The listing builds one solid part. Answer for the finished solid, in the listing's coordinates (mm). Round coordinates to 2 decimals unless told otherwise and drop trailing zeros. Write each loop counter-clockwise with the first axis right and the second up, starting at its lowest first coordinate (ties: lowest second). Pieces come first, ordered by that corner, then holes.
(1) A cutting plane is placed at D-D, the plane y = 1.75. Give the number of separate pieces and of enclosed holes in the cut face, and give its area (3 significant figures).
(2) A cutting plane is placed at B-B, the plane z = 0. Give the vertices of the cut face in (x, y).
(3) Find the intervals of material crossed by probe 1 along Z at (x, y) = (135.5, 7.5); probe 2 along X at (y, z) = (7, -6); probe 3 along X at (y, z) = (3.75, 270.5), in increasing order.
(4) The mould has two halves that part along X. Classify faces 1 (the face through (317.586, 4.93, -46.998)), 2 (the face through (-135.078, 4.93, -286.223)), 3 (the face through (-98, 10, 250)): +X half, -X half, draft (parallel to the pull), parting line (faces both ways), or undercut.
(5) Each of these flat-tipped pins is pushed along its axis until it touches: pin 1 Ø20.5 at (x, z) = (219.2, 219.2) entering from -Y; pin 2 Ø3 at (x, y) = (168.5, 8) entering from -Z; pin 3 Ø3 at (x, y) = (128, 1) entering from -Z. Where does it stop, or does it pass through?
(6) A cutting plane is placed at C-C, the plane x = 143. Give the vertices of the cut face in (y, z).
(7) A cutting plane is placed at A-A, the plane x = 0. Give the vertices of the cut face in (y, z), and give its area (3 significant figures).
Autodesk Inventor part; units mm, degrees
ref_plane "YZ Plane" through (0, 0, 0) normal (1, 0, 0) x (0, 1, 0)
ref_plane "XZ Plane" through (0, 0, 0) normal (0, 1, 0) x (-1, 0, 0)
ref_plane "XY Plane" through (0, 0, 0) normal (0, 0, 1) x (1, 0, 0)
sketch "Sketch1" plane through (0, 0, 0) normal (0, 1, 0) x (-1, 0, 0)
  circle A0 centre (0, 0) radius 266.5
  circle A1 centre (0, 0) radius 335
  line L0 (335, 0) -> (266.5, 0)
  line L1 (-266.5, 0) -> (-335, 0)
  line L2 (0, 266.5) -> (0, 335)
  point P0 (300.75, 0)
  point P1 (-300.75, 0)
  point P2 (0, 300.75)
  dimension "d1" = 670
  dimension "d4" = 533
extrude "Extrusion1" add sketch "Sketch1" along normal blind 10 contours L0 A1 L1 A0 | A0 L2 A1 L0 | A0 L1 A1 L2
sketch "Sketch2" plane through (0, 0, 0) normal (0, -1, 0) x (1, 0, 0)
  circle A0 centre (0, 0) radius 335
  circle A1 centre (0, 0) radius 266.5
  circle A2 centre (48.4947, 306.1834) radius 11.5
  circle A3 centre (0, 0) radius 266.5
  line L0 (48.4947, 306.1834) -> (0, 0)
  point P0 (0, 266.5)
  point P1 (265, 0)
  dimension "d5" = 310
  dimension "d7" = 23
extrude "Cut1" cut sketch "Sketch2" against normal blind 10 contours A2
pattern_circular "Circular Pattern1" count 20 over 360 about axis through (0, 0, 0) along (0, 1, 0) of "Cut1"
equation "\"d2\" = Thickness"
equation "\"d9\" = Thickness"
equation "\"BendReliefDepth\" = 0.5 * Thickness"
properties part number "PNS-612 accses hatch flangeipt_1200"
Solutions:
1. separate pieces: 1
1. enclosed holes: 21
1. area: 121,000 mm2
2. outline: (-335, 0) - (-266.5, 0) - (-266.5, 10) - (-335, 10) - close; (266.5, 0) - (335, 0) - (335, 10) - (266.5, 10) - close
3. probe 1: z = -306.37 to -286.45, -265.97 to -229.48, 229.48 to 265.97, 286.45 to 306.37
3. probe 2: x = -334.95 to -266.43, 266.43 to 334.95
3. probe 3: x = -197.62 to -150.72, -130.76 to 130.76, 150.72 to 197.62
4. face 1: undercut
4. face 2: undercut
4. face 3: draft
5. pin 1: passes through
5. pin 2: stops at z = -290.41
5. pin 3: stops at z = -310.2
6. outline: (0, -302.95) - (10, -302.95) - (10, -287.49) - (0, -287.49) - close; (0, -264.94) - (10, -264.94) - (10, -224.88) - (0, -224.88) - close; (0, 224.88) - (10, 224.88) - (10, 264.94) - (0, 264.94) - close; (0, 287.49) - (10, 287.49) - (10, 302.95) - (0, 302.95) - close
7. outline: (0, -335) - (10, -335) - (10, -266.5) - (0, -266.5) - close; (0, 266.5) - (10, 266.5) - (10, 335) - (0, 335) - close
7. area: 1,370 mm2
